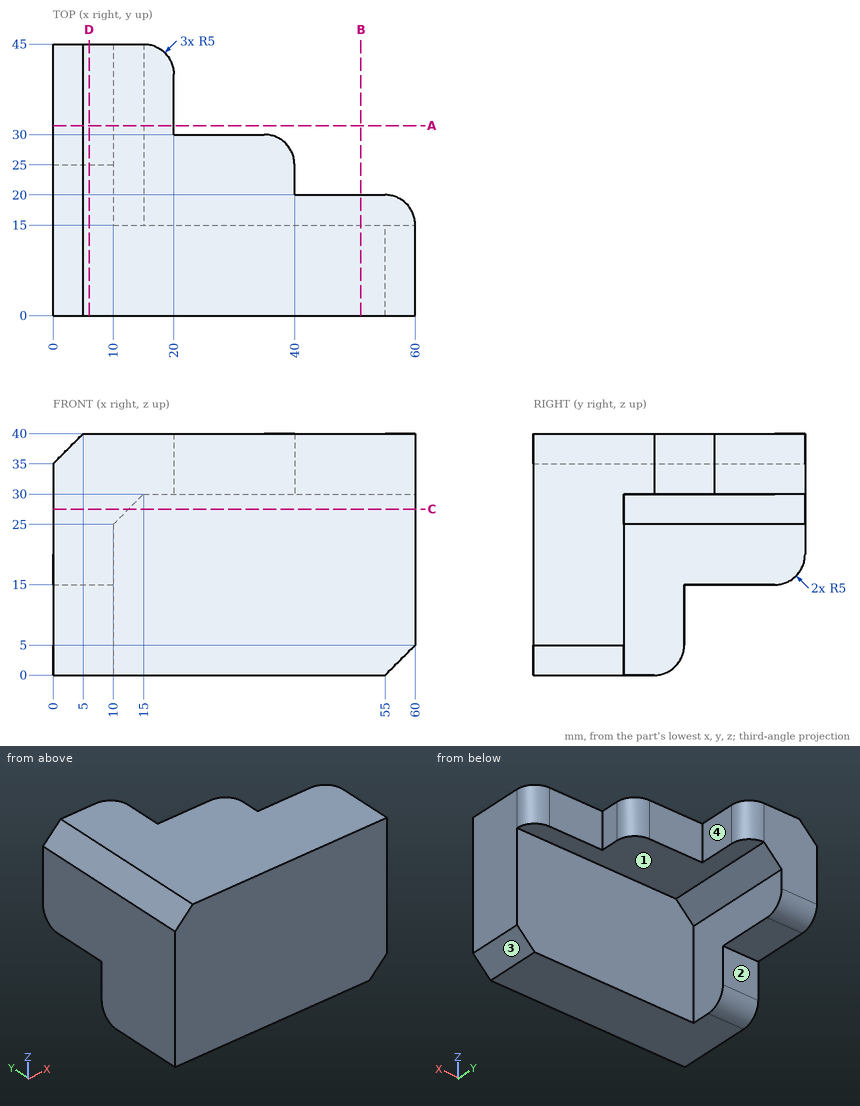
Source: three-view drawing plus pictorial views. Frame: mm from the lowest corner of the part. A direction names the side the tool comes from. Round coordinates to 2 decimals unless told otherwise and drop trailing zeros. Loops run counter-clockwise (first coordinate to the right, second up) from the corner with the lowest first, then second, coordinate; pieces in that order, holes last.
Q1. Section D-D, the plane x = 6. Return loops of the section in (y, z), plus the area to 3 significant figures.
Q2. First-contact query: P1, Ø24, axis at x = 28.5, z = 18.5, coming from the +Y side; P2, Ø5, axis at x = 14.5, z = 23, coming from the +Y side; P3, Ø3, axis at x = 3, z = 10.5, coming from the +Y side. Flat tips, straight axial feed; report the tip coordinate or a pass-through.
Q3. Section B-B, the plane x = 51. Return loops of the section in (y, z), plus the area to 3 significant figures.
Q4. Section C-C, the plane z = 27.5. Return loops of the section in (x, y), plus the area to 4 significant figures.
Q5. Ray query, line 1 (Y direction, x = 52, z = 26); line 2 (Z direction, x = 19.5, y = 42); line 3 (X direction, y = 27, z = 18). Return the intervals inside material, ascending.
Q6. Access query for the marked faces 1, 2, 3 and 4. Directions: +Z, -Z, +X, -X, +Y, -Y. A direction counts if a zero-diameter tool reaches every point of the face in a straight line with its end or side. Return the directions, or none.
Q7. Section A-A, the plane y = 31.5. Return loops of the section in (x, z).
Solutions:
1. outline: (0, 0) - (20, 0) arc R5 ccw to (25, 5) - (25, 15) - (40, 15) arc R5 ccw to (45, 20) - (45, 40) - (0, 40) - close
1. area: 1,490 mm2
2. P1: stops at y = 30
2. P2: stops at y = 15
2. P3: stops at y = 25
3. outline: (0, 0) - (15, 0) - (15, 30) - (20, 30) - (20, 40) - (0, 40) - close
3. area: 650 mm2
4. outline: (0, 0) - (60, 0) - (60, 15) - (12.5, 15) - (12.5, 45) - (0, 45) - close
4. area: 1,275 mm2
5. line 1: y = 0 to 15
5. line 2: z = 30 to 40
5. line 3: x = 0 to 10
6. face 1: -Z, +X, +Y
6. face 2: -Z, +X, -X, +Y
6. face 3: -Z, +X, +Y, -Y
6. face 4: +Z, -Z, +X, +Y
7. outline: (0, 15) - (10, 15) - (10, 25) - (15, 30) - (20, 30) - (20, 40) - (5, 40) - (0, 35) - close
